Build history of the part. All positions in model axes, mm. Give positions to 0.01 mm unless a question says otherwise; leave off trailing zeros. Loops run counter-clockwise (first coordinate to the right, second up) from the corner with the lowest first, then second, coordinate; pieces in that order, holes last. Notation, with made-up numbers: (-21.5, 89) -> (34.5, 89) arc R27 ccw to (34.5, 114) -> close; hole circle Ø3 at (40.5, 67). An arc over 180 degrees is marked (long way). Answer as a JSON object with one key per item and string values. Group by question number.
from build123d import *

# Parameters (mm, degrees)
F0_W     = 19.05
F0_H     = 88.9
F1_DEPTH = 304.8
F3_D     = 6.35
F5_DEPTH = 19.051


with BuildPart() as f1:
    # F0 (on Front) → F1 (new body)
    with BuildSketch(Plane.XZ):
        Rectangle(F0_W, F0_H)
    extrude(amount=F1_DEPTH)

    # F3 (through all)
    with Locations(Plane.YZ.offset(9.525)):
        with Locations((-44.45, 0)):
            Hole(F3_D / 2)

    # F4 (on face) → F5 (cut, through all)
    with BuildSketch(Plane.YZ.offset(9.525)):
        with BuildLine():
            Line((0, -44.45), (0, -0.568558))
            ThreePointArc((0, -0.568558), (-13.016533, -31.433467), (-43.881442, -44.45))
            Line((-43.881442, -44.45), (0, -44.45))
        make_face()
        with BuildLine():
            Line((0, 44.45), (-43.881442, 44.45))
            ThreePointArc((-43.881442, 44.45), (-13.016533, 31.433467), (0, 0.568558))
            Line((0, 0.568558), (0, 44.45))
        make_face()
    extrude(amount=-F5_DEPTH, mode=Mode.SUBTRACT)


solid = f1.part
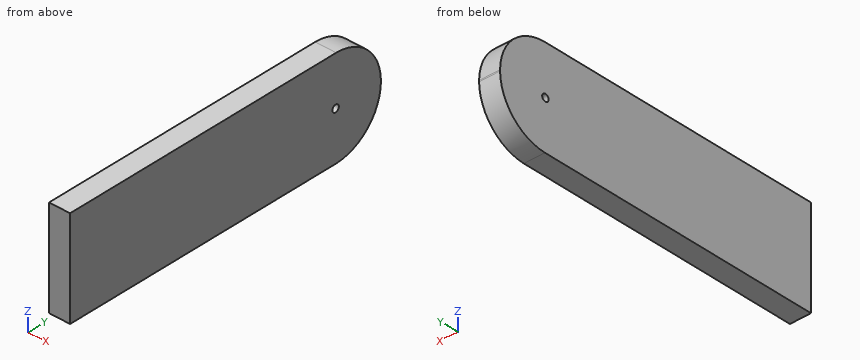
(1) Pin check, flat tip, straight feed: pin 1 (5 mm diameter, centred on y = -44.45, z = 0, fed in from +X). Stop position of the tip, or through.
(2) Probe line 1 along Z through (x, y) = (4.5, -44.45) (3 decimals); line 2 along Y through (x, z) = (-5.25, -27.5); line 3 along Y through (x, z) = (4, -7). List the from-to ranges inside material, lowest first. Write a range as [from, to].
(3) Saw through at A-A on x = 3.25. List the corners of the cut face in (y, z) (3 decimals), plus the area to 3 significant figures.
(4) Saw through at C-C on y = -19. List the corners of the cut face in (x, z) (3 decimals).
(5) Saw through at B-B on z = -31.5. List the corners of the cut face in (x, y) (3 decimals).
Calculated:
{
 "1": {"pin 1": "passes through"},
 "2": {"line 1": "z = [-44.45, -3.175], [3.175, 44.45]", "line 2": "y = [-304.8, -9.52]", "line 3": "y = [-304.8, -0.55]"},
 "3": {"outline": "(-304.8, -44.45) -> (-43.881, -44.45) arc R44.454 ccw to (0, -0.569) -> (0, 0.569) arc R44.454 ccw to (-43.881, 44.45) -> (-304.8, 44.45) -> close; hole circle Ø6.35 at (-44.45, 0)", "area": "26,200 mm^2"},
 "4": {"outline": "(-9.525, -36.448) -> (9.525, -36.448) -> (9.525, 36.448) -> (-9.525, 36.448) -> close"},
 "5": {"outline": "(-9.525, -304.8) -> (9.525, -304.8) -> (9.525, -13.083) -> (-9.525, -13.083) -> close"}
}
